Autodesk Inventor part; units mm, degrees
ref_plane "YZ Plane" through (0, 0, 0) normal (1, 0, 0) x (0, 1, 0)
ref_plane "XZ Plane" through (0, 0, 0) normal (0, 1, 0) x (-1, 0, 0)
ref_plane "XY Plane" through (0, 0, 0) normal (0, 0, 1) x (1, 0, 0)
sketch "Sketch1" plane through (0, 0, 0) normal (0, 1, 0) x (-1, 0, 0)
  line L0 (15, -35) -> (-15, -35)
  line L1 (-15, -35) -> (-15, 35)
  line L2 (-15, 35) -> (15, 35)
  line L3 (15, 35) -> (15, -35)
  line L4 (15, -35) -> (-15, 35) construction
  line L5 (-15, -35) -> (15, 35) construction
  point P0 (0, 0)
  dimension "d0" = 30
  dimension "d1" = 70
extrude "Extrusion1" add sketch "Sketch1" along normal blind 30
sketch "Sketch2" plane through (15, 0, 35) normal (1, 0, 0) x (0, 0, -1)
  circle A0 centre (35, 15.1375) radius 14.909
  line L0 (0, 0) -> (0, 30)
  line L1 (0, 8.8455) -> (70, 8.8455)
  line L2 (0, 30) -> (70, 30)
  line L3 (0, 0) -> (70, 0)
  line L4 (70, 0) -> (70, 30)
  point P0 (35, 0)
  point P1 (36.1767, 30)
  point P2 (21.4837, 8.8455)
  point P3 (33.8233, 30)
  point P4 (48.5163, 8.8455)
extrude "Extrusion2" cut sketch "Sketch2" against normal blind 30 contours A0 L2 L4 L1 | A0 L1 L0 L2
sketch "Sketch3" plane through (-15, 0, 35) normal (0, 0, 1) x (1, 0, 0)
  circle A0 centre (15, 19.3194) radius 10.5597
  line L0 (0, 30) -> (0, 8.8455)
  line L1 (0, 30) -> (30, 30)
  line L2 (30, 8.8455) -> (30, 30)
  line L3 (30, 8.8455) -> (0, 8.8455)
  point P0 (15, 0)
  point P1 (13.6563, 8.8455)
  point P2 (16.3437, 8.8455)
extrude "Extrusion3" cut sketch "Sketch3" against normal blind 77 contours A0 L3 L0 L1 L2
properties part number "ball transfer unit"
Here's how the part is built. I have some questions about the finished solid (model axes, mm). Coordinates: 2 decimals unless noted, no trailing zeros. Order: outer loops, then holes, each group sorted by start corner. A loop starts at its lowest first (then second) coordinate and runs counter-clockwise, first axis right, second up. Notation, with made-up numbers: (-32.75, 43) -> (16.25, 43) arc R16 cw to (16.25, 49) -> close; hole circle Ø2 at (2, 64). An arc over 180 degrees is marked (long way). Answer in a Markdown table with one row per item.
(1) I want a section at A-A on x = 0. List the corners of the cut face in (y, z) for me, then the cut area to 3 significant figures.
Answer key:
| item | result |
|---|---|
| outline | (0, -35) -> (8.85, -35) -> (8.85, -13.52) arc R14.91 ccw to (29.88, -2.23) -> (29.88, 2.23) arc R14.91 ccw to (8.85, 13.52) -> (8.85, 35) -> (0, 35) -> close |
| area | 1,150 mm^2 |
(2) Will these pins go through, and if not, where does the flat tip stop? pin 1 Ø1 at (y, z) = (11, 14.5) entering from -X; pin 2 Ø3 at (x, y) = (-4, 17) entering from -Z; pin 3 Ø2 at (x, z) = (-3, 3) entering from +Y.
Answer key:
| item | result |
|---|---|
| pin 1 | x = -7.09 |
| pin 2 | z = -14.9 |
| pin 3 | y = 29.69 |
(3) Thinking about a two-plate mould opening in Y: for faces 1 (the face through (0, 0, 0)), 2 (the face through (4.31, 9.68, 0.21)), 3 (the face through (4, 8.846, 0)), 4 (the face through (0, 4, 35)), which applies, +Y half, -Y half, draft (parallel to the pull), parting line (faces both ways), or undercut?
Answer key:
| item | result |
|---|---|
| face 1 | -Y half |
| face 2 | undercut |
| face 3 | undercut |
| face 4 | draft |
(4) I want a section at B-B on z = -24. List the corners of the cut face in (x, y) for me.
Answer key:
| item | result |
|---|---|
| outline | (-15, 0) -> (15, 0) -> (15, 8.85) -> (-15, 8.85) -> close |
(5) I want a section at C-C on y = 21.25. List the corners of the cut face in (x, z) for me.
Answer key:
| item | result |
|---|---|
| outline | (-10.38, -13.6) -> (10.38, -13.6) -> (10.38, 13.6) -> (-10.38, 13.6) -> close |
(6) Please list where these lines run through material, in increasing order: probe 1 along X at (y, z) = (19.25, -8.5); probe 2 along Y at (x, z) = (-9.75, -9.5); probe 3 along Y at (x, z) = (0, -27).
Answer key:
| item | result |
|---|---|
| probe 1 | -10.56 to 10.56 |
| probe 2 | 0 to 8.85, 15.26 to 23.37 |
| probe 3 | 0 to 8.85 |
